from build123d import *

# Parameters (mm, degrees)
SKETCH003_R  = 10
PAD003_DEPTH = 4
SKETCH001_R  = 3
PAD002_DEPTH = 10
PAD001_DEPTH = 35
PAD_DEPTH    = 42
FILLET_R     = 5


with BuildPart() as motormount:
    # Sketch003 → Pad003 (new body)
    with BuildSketch(Plane.XY.offset(13)):
        with Locations((-1.743039, 25.632756)):
            Circle(SKETCH003_R)
        with BuildLine():
            ThreePointArc((14.71762, 39.972094), (14.717625, 42.093413), (12.596306, 42.093421))
            Line((7.196308, 36.693422), (12.596306, 42.093421))
            ThreePointArc((7.196308, 36.693422), (7.196301, 34.572096), (9.317627, 34.572101))
            Line((9.317627, 34.572101), (14.71762, 39.972094))
        make_face()
        with BuildLine():
            ThreePointArc((12.596306, 9.172091), (14.717625, 9.172099), (14.71762, 11.293417))
            Line((9.317628, 16.693409), (14.71762, 11.293417))
            ThreePointArc((9.317628, 16.693409), (7.196301, 16.693416), (7.196308, 14.572089))
            Line((7.196308, 14.572089), (12.596306, 9.172091))
        make_face()
        with BuildLine():
            ThreePointArc((-16.082385, 42.093423), (-18.203705, 42.09341), (-18.203694, 39.972091))
            Line((-12.803692, 34.572088), (-18.203694, 39.972091))
            ThreePointArc((-12.803692, 34.572088), (-10.682372, 34.572101), (-10.682383, 36.693421))
            Line((-10.682383, 36.693421), (-16.082385, 42.093423))
        make_face()
        with BuildLine():
            ThreePointArc((-18.203691, 11.293424), (-18.203707, 9.172104), (-16.082386, 9.172087))
            Line((-16.082386, 9.172087), (-10.682386, 14.572088))
            ThreePointArc((-10.682386, 14.572088), (-10.68237, 16.693408), (-12.80369, 16.693424))
            Line((-18.203691, 11.293424), (-12.80369, 16.693424))
        make_face()
    extrude(amount=-PAD003_DEPTH)


with BuildPart() as cutblock:
    # Sketch001 → Pad002 (new body)
    with BuildSketch(Plane(origin=(0, 5.632756, 0), x_dir=(-1, 0, 0), z_dir=(0, 1, 0))):
        with Locations((-16.256961, 23)):
            Circle(SKETCH001_R)
        with Locations((19.743039, 23)):
            Circle(SKETCH001_R)
    extrude(amount=-PAD002_DEPTH)

    # Fusion001: union MotorMount
    add(motormount.part)


with BuildPart() as base:
    # Sketch → Pad001 (new body)
    with BuildSketch(Plane.XY):
        with BuildLine():
            Line((-31.743039, 5.632756), (28.256961, 5.632756))
            Line((28.256961, 5.632756), (28.256961, -4.367244))
            Line((2.256961, -4.367244), (28.256961, -4.367244))
            ThreePointArc((2.256961, -4.367244), (-1.743039, -0.367244), (-5.743039, -4.367244))
            Line((-31.743039, -4.367244), (-5.743039, -4.367244))
            Line((-31.743039, -4.367244), (-31.743039, 5.632756))
        make_face()
    extrude(amount=PAD001_DEPTH)


with BuildPart() as fillet_body:
    # Sketch002 → Pad (new body)
    with BuildSketch(Plane(origin=(0, 5.632756, 0), x_dir=(-1, 0, 0), z_dir=(0, 1, 0))):
        Polygon((-24.256961, 13), (27.743039, 13), (27.743039, 0), (22.843039, 0), (22.843039, 9), (-19.356961, 9), (-19.356961, 0), (-24.256961, 0), align=None)
    extrude(amount=PAD_DEPTH)

    # Fusion: union Base
    add(base.part)

    # Cut: cut CutBlock
    add(cutblock.part, mode=Mode.SUBTRACT)

    # Fillet
    fillet_edges = [fillet_body.edges().sort_by_distance(p)[0] for p in [
        (-1.743039, 5.632756, 35),
    ]]
    fillet(fillet_edges, radius=FILLET_R)


solid = fillet_body.part
For this review, take the finished solid that the model builds, in its own axes (mm). A direction names the side the tool comes from. Round coordinates to 2 decimals unless told otherwise and drop trailing zeros. Order: outer loops, then holes, each group sorted by start corner. A loop starts at its lowest first (then second) coordinate and runs counter-clockwise, first axis right, second up. Notation, with made-up numbers: (45.25, -26.75) -> (90.25, -26.75) arc R17 cw to (90.25, -4.75) -> close; hole circle Ø2 at (-13, -16.5). An arc over 180 degrees is marked (long way). Write item = value, one per line. Start each with the question number.
1) Take a section at C-C on y = 31.5. State the section outline as (x, z) points, plus the area to 3 significant figures.
2) Take a section at A-A on z = 23. State the section outline as (x, y) points, plus the area to 3 significant figures.
3) Tool access review of faces 5 (the face through (-27.743, 26, 7)), 6 (the face through (9.86, 11.91, 11.03)), 7 (the face through (24.257, 26, 6)), 8 (the face through (19.357, 26, 5)): name each direction out of +Z, -Z, +X, -X, +Y, -Y from which nothing blocks a thin tool from reaching the whole face with its end or side.
4) Insertion check: pin 1 (4.5 mm diameter, centred on x = -10, z = 3.5, fed in from +Y); pin 2 (2 mm diameter, centred on y = 9.5, z = 8.5, fed in from +X); pin 3 (21 mm diameter, centred on x = -11.5, y = 24, fed in from +Z); pin 4 (7 mm diameter, centred on x = 16.26, z = 23, fed in from -Y). Each pin has a flat end and moves straight along its axis. Give the tip position at first contact, or say it passes through.
5) Take a section at D-D on x = -14.5. State the section outline as (y, z) points.
6) Take a section at B-B on x = -24.5. State the section outline as (y, z) points, plus the area to 3 significant figures.
7) The part is to be moulded in two halves that separate along Z. For faces 1 (the face through (-1, 0, 35)), 2 (the face through (19.254, 0.703, 23.132)), 3 (the face through (-2, 36, 9)), 4 (the face through (-18, 9, 11)), say which applies: +Z half, -Z half, draft (parallel to the pull), parting line (faces both ways), or undercut.
8) To check wall thickness, follow line 1 (X direction, y = 44.5, z = 6); line 2 (Z direction, x = 19, y = 34.5); line 3 (Z direction, x = -27, y = 45). State the ranges of each line that lie inside material, in increasing order. Write a range as from..to.
Verdict:
q1.outline = (-27.74, 0) -> (-22.84, 0) -> (-22.84, 9) -> (-9.84, 9) -> (-9.84, 13) -> (-27.74, 13) -> close; (6.35, 9) -> (19.36, 9) -> (19.36, 0) -> (24.26, 0) -> (24.26, 13) -> (6.35, 13) -> close
q1.area = 231 mm2
q2.outline = (-31.74, -4.37) -> (-22.74, -4.37) -> (-22.74, 5.63) -> (-31.74, 5.63) -> close; (-16.74, -4.37) -> (-5.74, -4.37) arc R4 cw to (2.26, -4.37) -> (13.26, -4.37) -> (13.26, 5.63) -> (-16.74, 5.63) -> close; (19.26, -4.37) -> (28.26, -4.37) -> (28.26, 5.63) -> (19.26, 5.63) -> close
q2.area = 455 mm2
q3.face_5 = +Z, -Z, -X, +Y
q3.face_6 = +Z, -Z
q3.face_7 = +Z, -Z, +X, +Y
q3.face_8 = -Z, +Y
q4.pin_1 = 5.63
q4.pin_2 = 24.26
q4.pin_3 = 13
q4.pin_4 = -4.37
q5.outline = (-4.37, 0) -> (5.63, 0) -> (5.63, 9) -> (10.75, 9) -> (10.75, 13) -> (5.63, 13) -> (5.63, 30) arc R5 ccw to (0.63, 35) -> (-4.37, 35) -> close; (15, 9) -> (36.27, 9) -> (36.27, 13) -> (15, 13) -> close; (40.51, 9) -> (47.63, 9) -> (47.63, 13) -> (40.51, 13) -> close
q6.outline = (-4.37, 0) -> (47.63, 0) -> (47.63, 13) -> (5.63, 13) -> (5.63, 30) arc R5 ccw to (0.63, 35) -> (-4.37, 35) -> close
q6.area = 891 mm2
q7.face_1 = +Z half
q7.face_2 = undercut
q7.face_3 = -Z half
q7.face_4 = draft
q8.line_1 = -27.74..-22.84, 19.36..24.26
q8.line_2 = 9..13
q8.line_3 = 0..13
